Autodesk Inventor part; units mm, degrees
ref_plane "Arbeitsebene3" through (-32.75, 5, -38) normal (0, 1, 0) x (0, 0, 1)
ref_plane "YZ Plane" through (0, 0, 0) normal (1, 0, 0) x (0, 1, 0)
ref_plane "XZ Plane" through (0, 0, 0) normal (0, 1, 0) x (-1, 0, 0)
sketch "Skizze1" plane through (0, 0, 0) normal (0, 1, 0) x (-1, 0, 0)
  line L0 (-37.75, -63.9) -> (37.75, -63.9)
  line L1 (42.75, -58.9) -> (42.75, 58.9)
  line L2 (37.75, 63.9) -> (-37.75, 63.9)
  line L3 (-42.75, 58.9) -> (-42.75, -58.9)
  line L4 (-42.75, -63.9) -> (42.75, 63.9) construction
  line L5 (42.75, -63.9) -> (-42.75, 63.9) construction
  arc A0 (42.75, 58.9) -> (37.75, 63.9) centre (37.75, 58.9) ccw
  arc A1 (-37.75, 63.9) -> (-42.75, 58.9) centre (-37.75, 58.9) ccw
  arc A2 (-42.75, -58.9) -> (-37.75, -63.9) centre (-37.75, -58.9) ccw
  arc A3 (37.75, -63.9) -> (42.75, -58.9) centre (37.75, -58.9) ccw
  point P0 (0, 0)
  dimension "d0" = 85.5
  dimension "d1" = 127.8
  dimension "d2" = 5
extrude "Extrusion1" add sketch "Skizze1" along normal blind 10
ref_plane "Arbeitsebene1" through (37.75, 0, 0) normal (0, 0, -1) x (-1, 0, 0)
ref_plane "Arbeitsebene2" through (0, 0, 58.9) normal (1, 0, 0) x (0, 0, -1)
sketch "Skizze2" plane through (0, 10, 0) normal (0, 1, 0) x (1, 0, 0)
  line L0 (-6.95, 38) -> (-32.75, 38)
  line L1 (-32.75, -38) -> (-6.95, -38)
  line L2 (-6.95, -38) -> (-6.95, -2.5)
  line L3 (-32.75, 38) -> (-32.75, -38)
  line L4 (-32.75, -38) -> (-6.95, -38)
  line L5 (-6.95, -38) -> (-6.95, 38)
  line L6 (-6.95, 38) -> (-32.75, 38)
  line L7 (-32.75, 38) -> (-32.75, -38)
  line L8 (-5.95, 39) -> (-5.95, -39)
  line L9 (-5.95, -39) -> (-33.75, -39)
  line L10 (-33.75, -39) -> (-33.75, 39)
  line L11 (-33.75, 39) -> (-5.95, 39)
  point P0 (0, 0)
  dimension "d5" = 1
extrude "Extrusion2" cut sketch "Skizze2" against normal through all contours L5 L2 L1 L3 L0 | L8 L9 L10 L11
ref_plane "Arbeitsebene3" through (-32.75, 5, -38) normal (0, 1, 0) x (0, 0, 1)
sketch "Skizze3" plane through (0, 10, 0) normal (0, 1, 0) x (1, 0, 0)
  line L0 (-5.95, -39) -> (-33.75, -39)
  line L1 (-33.75, -39) -> (-33.75, 39)
  line L2 (-33.75, 39) -> (-5.95, 39)
  line L3 (-5.95, 39) -> (-5.95, -39)
  arc A0 (-37.75, 63.9) -> (-42.75, 58.9) centre (-37.75, 58.9) ccw
  line L4 (-42.75, 58.9) -> (-42.75, -58.9)
  arc A1 (-42.75, -58.9) -> (-37.75, -63.9) centre (-37.75, -58.9) ccw
  line L5 (-37.75, -63.9) -> (37.75, -63.9)
  arc A2 (37.75, -63.9) -> (42.75, -58.9) centre (37.75, -58.9) ccw
  line L6 (42.75, -58.9) -> (42.75, 58.9)
  arc A3 (42.75, 58.9) -> (37.75, 63.9) centre (37.75, 58.9) ccw
  line L7 (37.75, 63.9) -> (-37.75, 63.9)
  line L8 (-33.75, -39) -> (-33.75, 39)
  line L9 (-5.95, 39) -> (-5.95, -39)
  line L10 (-33.75, -39) -> (-5.95, -39)
  line L11 (-5.95, -39) -> (-5.95, -34)
  line L12 (-5.95, -34) -> (-33.75, -34)
  line L13 (-33.75, -34) -> (-33.75, -39)
  line L14 (-33.75, 39) -> (-5.95, 39)
  line L15 (-5.95, 39) -> (-5.95, 34)
  line L16 (-5.95, 34) -> (-33.75, 34)
  line L17 (-33.75, 34) -> (-33.75, 39)
  point P0 (0, 0)
  point P1 (-5.95, 34)
  point P2 (-5.95, -34)
  dimension "d8" = 27.8
  dimension "d9" = 5
  dimension "d10" = 5
extrude "Extrusion3" add sketch "Skizze3" against normal blind 1 contours L0 L1 L12 L3 | L16 L1 L2 L3
sketch "Skizze4" plane through (0, 0, 0) normal (0, -1, 0) x (1, 0, 0)
  line L0 (-33.75, 39) -> (-5.95, 39)
  line L1 (-5.95, 39) -> (-5.95, -39)
  line L2 (-5.95, -39) -> (-33.75, -39)
  line L3 (-33.75, -39) -> (-33.75, 39)
  arc A0 (-42.75, -58.9) -> (-37.75, -63.9) centre (-37.75, -58.9) ccw
  line L4 (37.75, -63.9) -> (-37.75, -63.9)
  arc A1 (37.75, -63.9) -> (42.75, -58.9) centre (37.75, -58.9) ccw
  line L5 (42.75, 58.9) -> (42.75, -58.9)
  arc A2 (42.75, 58.9) -> (37.75, 63.9) centre (37.75, 58.9) ccw
  line L6 (-37.75, 63.9) -> (37.75, 63.9)
  arc A3 (-37.75, 63.9) -> (-42.75, 58.9) centre (-37.75, 58.9) ccw
  line L7 (-42.75, -58.9) -> (-42.75, 58.9)
  line L8 (-5.95, -34) -> (-5.95, 34)
  line L9 (-5.95, 34) -> (21.3958, 34)
  line L10 (21.3958, 34) -> (21.3958, -34)
  line L11 (21.3958, -34) -> (-5.95, -34)
  line L12 (-5.95, -34) -> (-5.95, 34)
  line L13 (3.55, 7.5) -> (3.55, -8)
  point P0 (0, 0)
  point P1 (-5.95, -34)
  dimension "d14" = 5
  dimension "d15" = 5
extrude "Extrusion4" cut sketch "Skizze4" against normal through all contours L9 L10 L11 L1
sketch "Skizze5" plane through (0, 0, 0) normal (0, -1, 0) x (1, 0, 0)
  arc A0 (-42.75, -58.9) -> (-37.75, -63.9) centre (-37.75, -58.9) ccw
  line L0 (37.75, -63.9) -> (-37.75, -63.9)
  arc A1 (37.75, -63.9) -> (42.75, -58.9) centre (37.75, -58.9) ccw
  line L1 (42.75, 58.9) -> (42.75, -58.9)
  arc A2 (42.75, 58.9) -> (37.75, 63.9) centre (37.75, 58.9) ccw
  line L2 (-37.75, 63.9) -> (37.75, 63.9)
  arc A3 (-37.75, 63.9) -> (-42.75, 58.9) centre (-37.75, 58.9) ccw
  line L3 (-42.75, -58.9) -> (-42.75, 58.9)
  line L4 (-5.95, 34) -> (21.3958, 34)
  line L5 (21.3958, 34) -> (21.3958, -34)
  line L6 (21.3958, -34) -> (-5.95, -34)
  line L7 (-5.95, -34) -> (-5.95, -39)
  line L8 (-5.95, -39) -> (-33.75, -39)
  line L9 (-33.75, -39) -> (-33.75, 39)
  line L10 (-33.75, 39) -> (-5.95, 39)
  line L11 (-5.95, 39) -> (-5.95, 34)
  circle A4 centre (-19.85, -47) radius 1.4
  circle A5 centre (-19.85, 47) radius 1.4
  point P0 (0, 0)
  dimension "d18" = 2.8
  dimension "d19" = 2.8
  dimension "d20" = 8
  dimension "d21" = 8
extrude "Extrusion5" cut sketch "Skizze5" against normal through all contours A4 | A5
sketch "Skizze6" plane through (0, 10, 0) normal (0, 1, 0) x (1, 0, 0)
  circle A0 centre (25.45, -17.36) radius 1.57
  circle A1 centre (32.55, -17.36) radius 1.57
  circle A2 centre (32.55, 29.54) radius 1.57
  circle A3 centre (25.45, 29.54) radius 1.57
  line L0 (21.45, 51.1) -> (36.55, 51.1)
  line L1 (36.55, 42.04) -> (36.55, 51.1)
  line L2 (34.55, 42.04) -> (36.55, 42.04)
  line L3 (34.55, 34.04) -> (34.55, 42.04)
  line L4 (36.55, 34.04) -> (34.55, 34.04)
  line L5 (36.55, -21.86) -> (36.55, 34.04)
  line L6 (36.55, -21.86) -> (34.55, -21.86)
  line L7 (34.55, -21.86) -> (34.55, -29.86)
  line L8 (34.55, -29.86) -> (36.55, -29.86)
  line L9 (36.55, -29.86) -> (36.55, -38.92)
  line L10 (36.55, -38.92) -> (21.45, -38.92)
  line L11 (21.45, -38.92) -> (21.45, -29.86)
  line L12 (21.45, -29.86) -> (23.45, -29.86)
  line L13 (23.45, -29.86) -> (23.45, -21.86)
  line L14 (23.45, -21.86) -> (21.45, -21.86)
  line L15 (21.45, -21.86) -> (21.45, 34.04)
  line L16 (23.45, 34.04) -> (21.45, 34.04)
  line L17 (23.45, 42.04) -> (23.45, 34.04)
  line L18 (21.45, 42.04) -> (23.45, 42.04)
  line L19 (21.45, 51.1) -> (21.45, 42.04)
  circle A4 centre (25.45, 29.54) radius 1.57
  circle A5 centre (32.55, 29.54) radius 1.57
  circle A6 centre (25.45, -17.36) radius 1.57
  circle A7 centre (32.55, -17.36) radius 1.57
  circle A8 centre (21.9, 29.54) radius 1.57
  circle A9 centre (29, 29.54) radius 1.57
  circle A10 centre (21.9, -17.36) radius 1.57
  circle A11 centre (29, -17.36) radius 1.57
  point P0 (0, 0)
hole "Bohrung1" at (29, 10, 17.36) at (29, 10, -29.54) at (21.9, 10, -29.54) at (21.9, 10, 17.36) direction (0, -1, 0) diameter 4 end through all counterbore diameter 7 counterbore depth 4
sketch "Skizze7" plane through (21.9, 6, -29.54) normal (0, 1, 0) x (1, 0, 0)
  circle A0 centre (7.1, 0) radius 2
  arc A1 (-0.5042, -1.9354) -> (-0.5042, 1.9354) centre (0, 0) ccw
  line L0 (9.2, -49.54) -> (5, -49.54)
  circle A2 centre (7.1, -46.9) radius 2
  arc A3 (-0.5042, -48.8354) -> (-0.5042, -44.9646) centre (0, -46.9) ccw
  arc A4 (-0.5042, -50.3635) -> (-0.5042, -43.4365) centre (0, -46.9) ccw
  line L1 (0, -46.9) -> (10.0593, -46.9) construction
  line L2 (0, -44.9) -> (10.0593, -44.9)
  line L3 (10.0593, -48.9) -> (0, -48.9)
  arc A5 (0, -44.9) -> (0, -48.9) centre (0, -46.9) ccw
  arc A6 (10.0593, -48.9) -> (10.0593, -44.9) centre (10.0593, -46.9) ccw
  arc A7 (-0.5042, -1.9354) -> (-0.5042, 1.9354) centre (0, 0) ccw
  line L4 (0, 0) -> (10.0593, 0) construction
  line L5 (0, 2) -> (10.0593, 2)
  line L6 (10.0593, -2) -> (0, -2)
  arc A8 (0, 2) -> (0, -2) centre (0, 0) ccw
  arc A9 (10.0593, -2) -> (10.0593, 2) centre (10.0593, 0) ccw
  point P0 (-21.9, -29.54)
  point P1 (5.0296, -46.9)
  point P2 (5.0296, 0)
  point P3 (0, -48.9)
  point P4 (0, -2)
  point P5 (0, 2)
extrude "Extrusion6" cut sketch "Skizze7" against normal through all
sketch "Skizze8" plane through (0, 10, 0) normal (0, 1, 0) x (1, 0, 0)
  arc A0 (21.3958, 26.0765) -> (21.3958, 33.0035) centre (21.9, 29.54) ccw
  line L0 (21.3958, 26.0765) -> (21.3958, -13.8965)
  arc A1 (21.3958, -20.8235) -> (21.3958, -13.8965) centre (21.9, -17.36) ccw
  line L1 (21.3958, -20.8235) -> (21.3958, -34)
  line L2 (21.3958, -34) -> (-33.75, -34)
  line L3 (-33.75, -34) -> (-33.75, 34)
  line L4 (-33.75, 34) -> (21.3958, 34)
  line L5 (21.3958, 34) -> (21.3958, 33.0035)
  circle A2 centre (29, -17.36) radius 3.5
  circle A3 centre (29, 29.54) radius 3.5
  circle A4 centre (-19.85, -47) radius 1.4
  circle A5 centre (-19.85, 47) radius 1.4
  arc A6 (-37.75, 63.9) -> (-42.75, 58.9) centre (-37.75, 58.9) ccw
  line L6 (-42.75, 58.9) -> (-42.75, -58.9)
  arc A7 (-42.75, -58.9) -> (-37.75, -63.9) centre (-37.75, -58.9) ccw
  line L7 (-37.75, -63.9) -> (37.75, -63.9)
  arc A8 (37.75, -63.9) -> (42.75, -58.9) centre (37.75, -58.9) ccw
  line L8 (42.75, -58.9) -> (42.75, 58.9)
  arc A9 (42.75, 58.9) -> (37.75, 63.9) centre (37.75, 58.9) ccw
  line L9 (37.75, 63.9) -> (-37.75, 63.9)
  arc A10 (21.3958, 26.0765) -> (21.3958, 33.0035) centre (21.9, 29.54) ccw
  line L10 (21.9, 29.54) -> (34.3149, 29.54) construction
  line L11 (21.9, 26.04) -> (34.3149, 26.04)
  line L12 (34.3149, 33.04) -> (21.9, 33.04)
  arc A11 (21.9, 33.04) -> (21.9, 26.04) centre (21.9, 29.54) ccw
  arc A12 (34.3149, 26.04) -> (34.3149, 33.04) centre (34.3149, 29.54) ccw
  line L13 (21.9, -17.36) -> (34.3149, -17.36) construction
  line L14 (21.9, -20.86) -> (34.3149, -20.86)
  line L15 (34.3149, -13.86) -> (21.9, -13.86)
  arc A13 (21.9, -13.86) -> (21.9, -20.86) centre (21.9, -17.36) ccw
  arc A14 (34.3149, -20.86) -> (34.3149, -13.86) centre (34.3149, -17.36) ccw
  point P0 (0, 0)
  point P1 (28.1075, 29.54)
  point P2 (28.1075, -17.36)
  point P3 (21.3958, -13.8965)
  point P4 (21.3958, 33.0035)
extrude "Extrusion7" cut sketch "Skizze8" against normal up to surface (4 mm away) contours A11 A0 | A0 L12 A3 L11 | A1 A13 | A3 | A3 L12 A12 L11 | L15 A2 L14 A1 | L15 A14 L14 A2 | A2
sketch "Skizze9" plane through (0, 9, 0) normal (0, -1, 0) x (1, 0, 0)
  circle A0 centre (-19.85, 47) radius 1.4
  circle A1 centre (-19.85, -47) radius 1.4
  arc A2 (-42.75, -58.9) -> (-37.75, -63.9) centre (-37.75, -58.9) ccw
  line L0 (37.75, -63.9) -> (-37.75, -63.9)
  arc A3 (37.75, -63.9) -> (42.75, -58.9) centre (37.75, -58.9) ccw
  line L1 (42.75, 58.9) -> (42.75, -58.9)
  arc A4 (42.75, 58.9) -> (37.75, 63.9) centre (37.75, 58.9) ccw
  line L2 (-37.75, 63.9) -> (37.75, 63.9)
  arc A5 (-37.75, 63.9) -> (-42.75, 58.9) centre (-37.75, 58.9) ccw
  line L3 (-42.75, -58.9) -> (-42.75, 58.9)
  line L4 (21.9, 19.36) -> (31.9593, 19.36)
  arc A6 (31.9593, 15.36) -> (31.9593, 19.36) centre (31.9593, 17.36) ccw
  line L5 (31.9593, 15.36) -> (21.9, 15.36)
  arc A7 (21.3958, 15.4246) -> (21.9, 15.36) centre (21.9, 17.36) ccw
  line L6 (21.3958, 15.4246) -> (21.3958, -27.6046)
  arc A8 (21.9, -27.54) -> (21.3958, -27.6046) centre (21.9, -29.54) ccw
  line L7 (21.9, -27.54) -> (31.9593, -27.54)
  arc A9 (31.9593, -31.54) -> (31.9593, -27.54) centre (31.9593, -29.54) ccw
  line L8 (31.9593, -31.54) -> (21.9, -31.54)
  arc A10 (21.3958, -31.4754) -> (21.9, -31.54) centre (21.9, -29.54) ccw
  line L9 (21.3958, -31.4754) -> (21.3958, -34)
  line L10 (21.3958, -34) -> (-5.95, -34)
  line L11 (-5.95, -34) -> (-5.95, -39)
  line L12 (-5.95, -39) -> (-33.75, -39)
  line L13 (-33.75, -39) -> (-33.75, 39)
  line L14 (-33.75, 39) -> (-5.95, 39)
  line L15 (-5.95, 39) -> (-5.95, 34)
  line L16 (-5.95, 34) -> (21.3958, 34)
  line L17 (21.3958, 34) -> (21.3958, 19.2954)
  arc A11 (21.9, 19.36) -> (21.3958, 19.2954) centre (21.9, 17.36) ccw
  line L18 (-33.75, 39) -> (-5.95, 39)
  line L19 (-33.75, 39) -> (-5.95, 39)
  line L20 (-5.95, 39) -> (-5.95, 34)
  line L21 (-5.95, 34) -> (-33.75, 34)
  line L22 (-33.75, 34) -> (-33.75, 39)
  line L23 (-5.95, -39) -> (-33.75, -39)
  line L24 (-33.75, -39) -> (-33.75, -34)
  line L25 (-5.95, -39) -> (-33.75, -39)
  line L26 (-33.75, -39) -> (-33.75, -34)
  line L27 (-33.75, -34) -> (-5.95, -34)
  line L28 (-5.95, -34) -> (-5.95, -39)
  point P0 (0, 0)
extrude "Extrusion8" add sketch "Skizze9" along normal blind 1 contours L21 L13 L14 L15 | L27 L11 L12 L13
properties part number "TIRFImager_base_v0"
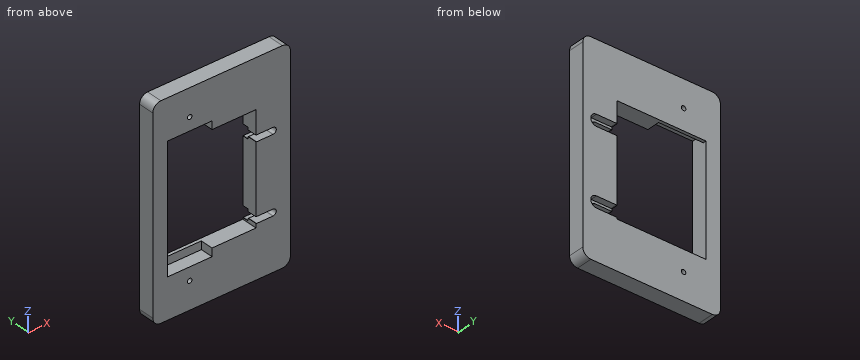
Work out the finished part from the listing and answer in its coordinate system (mm). Give positions to 0.01 mm unless a question says otherwise; leave off trailing zeros. Loops run counter-clockwise (first coordinate to the right, second up) from the corner with the lowest first, then second, coordinate; pieces in that order, holes last. Notation, with made-up numbers: (-11.75, -38.5) -> (19.25, -38.5) arc R16 ccw to (19.25, -31.5) -> close; hole circle Ø8 at (14, 66.25). An arc over 180 degrees is marked (long way). Use a Markdown table: item, result. Add a question column.
1. Find the intervals of material crossed by probe 1 along Z at (x, y) = (-19.85, 2.5); probe 2 along Z at (x, y) = (30, 0.5); probe 3 along Z at (x, y) = (0.5, 4.75), in increasing order.
2. Section B-B on x = 23.5 is taken. Determine the outline of the cut face in (y, z).
3. Section A-A on x = -19.85 is taken. Determine the outline of the cut face in (y, z), and give its area (3 significant figures).
4. Flat-ended cylindrical pins translate along their axes: pin 1 Ø4 at (x, z) = (-26.5, -36) entering from -Y; pin 2 Ø10 at (x, z) = (-1.5, 50) entering from -Y; pin 3 Ø2.5 at (x, z) = (-19.85, -47) entering from +Y. Find the tip coordinate at first contact, or state that the pin passes through.
5. Section C-C on z = -5.5 is taken. Determine the outline of the cut face in (x, y), and give its area (3 significant figures).
6. Section D-D on x = 13 is taken. Determine the outline of the cut face in (y, z), and give its area (3 significant figures).
Results below:
| question | item | result |
|---|---|---|
| 1 | probe 1 | z = -63.9 to -48.4, -45.6 to -39, 39 to 45.6, 48.4 to 63.9 |
| 1 | probe 2 | z = -63.9 to -31.54, -27.54 to 15.36, 19.36 to 63.9 |
| 1 | probe 3 | z = -63.9 to -34, 34 to 63.9 |
| 2 | outline | (0, -63.9) -> (10, -63.9) -> (10, -33.04) -> (6, -33.04) -> (6, -31.54) -> (0, -31.54) -> close; (0, -27.54) -> (6, -27.54) -> (6, -26.04) -> (10, -26.04) -> (10, 13.86) -> (6, 13.86) -> (6, 15.36) -> (0, 15.36) -> close; (0, 19.36) -> (6, 19.36) -> (6, 20.86) -> (10, 20.86) -> (10, 63.9) -> (0, 63.9) -> close |
| 3 | outline | (0, -63.9) -> (10, -63.9) -> (10, -48.4) -> (0, -48.4) -> close; (0, -45.6) -> (10, -45.6) -> (10, -34) -> (8, -34) -> (8, -39) -> (0, -39) -> close; (0, 39) -> (8, 39) -> (8, 34) -> (10, 34) -> (10, 45.6) -> (0, 45.6) -> close; (0, 48.4) -> (10, 48.4) -> (10, 63.9) -> (0, 63.9) -> close |
| 3 | area | 462 mm^2 |
| 4 | pin 1 | stops at y = 8 |
| 4 | pin 2 | stops at y = 0 |
| 4 | pin 3 | passes through |
| 5 | outline | (-42.75, 0) -> (-33.75, 0) -> (-33.75, 10) -> (-42.75, 10) -> close; (21.4, 0) -> (42.75, 0) -> (42.75, 10) -> (21.4, 10) -> close |
| 5 | area | 304 mm^2 |
| 6 | outline | (0, -63.9) -> (10, -63.9) -> (10, -34) -> (0, -34) -> close; (0, 34) -> (10, 34) -> (10, 63.9) -> (0, 63.9) -> close |
| 6 | area | 598 mm^2 |
